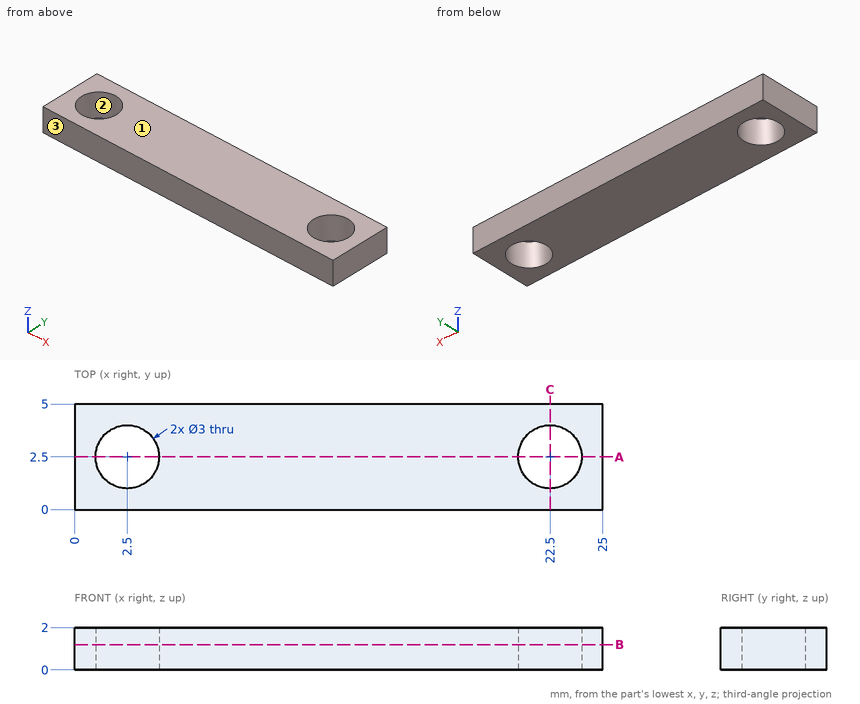
Can you work these out from the drawing? Everything is in mm from the part's minimum corner. Give positions to 0.01 mm unless a question says otherwise; leave off trailing zeros. Loops run counter-clockwise (first coordinate to the right, second up) from the corner with the lowest first, then second, coordinate; pieces in that order, holes last. Notation, with made-up numbers: (68.25, 12) -> (83.25, 12) arc R16 cw to (83.25, 21) -> close; hole circle Ø11 at (50, 81). An arc over 180 degrees is marked (long way). Return JSON: item names as keys, results as strings.
Q1. I need wall thicknesses on probe 1 along X at (y, z) = (2.5, 1); probe 2 along X at (y, z) = (1.25, 1.75); probe 3 along Y at (x, z) = (22.5, 0.6). Which ranges of each line are inside material? Lowest first, please.
Checks:
{"probe 1": "x = 0 to 1, 4 to 21, 24 to 25", "probe 2": "x = 0 to 1.67, 3.33 to 21.67, 23.33 to 25", "probe 3": "y = 0 to 1, 4 to 5"}
Q2. I want a section at C-C, the plane x = 22.5. List the corners of the cut face in (y, z) for me.
Checks:
{"outline": "(0, 0) -> (1, 0) -> (1, 2) -> (0, 2) -> close; (4, 0) -> (5, 0) -> (5, 2) -> (4, 2) -> close"}
Q3. We'd pull the mould along Y, two halves only. Please class the marked faces 1, 2 and 3: released by +Y, released by -Y, zero draft, split by the parting line, or undercut.
Checks:
{"face 1": "zero draft", "face 2": "undercut", "face 3": "released by -Y"}
Q4. For pin 1 Ø1.5 at (x, y) = (22, 3) entering from +Z, with a flat end and sliding along its axis, tell me the tip position at first contact or that it passes through.
Checks:
{"pin 1": "passes through"}
Q5. I want a section at B-B, the plane z = 1.2. List the corners of the cut face in (x, y) for me.
Checks:
{"outline": "(0, 0) -> (25, 0) -> (25, 5) -> (0, 5) -> close; hole circle Ø3 at (2.5, 2.5); hole circle Ø3 at (22.5, 2.5)"}
Q6. I want a section at A-A, the plane y = 2.5. List the corners of the cut face in (x, z) for me.
Checks:
{"outline": "(0, 0) -> (1, 0) -> (1, 2) -> (0, 2) -> close; (4, 0) -> (21, 0) -> (21, 2) -> (4, 2) -> close; (24, 0) -> (25, 0) -> (25, 2) -> (24, 2) -> close"}
